Work out the finished part from the listing and answer in its coordinate system (mm). A direction names the side the tool comes from. Round coordinates to 2 decimals unless told otherwise and drop trailing zeros. Write each loop counter-clockwise with the first axis right and the second up, starting at its lowest first coordinate (ties: lowest second). Pieces come first, ordered by that corner, then holes.
1. Determine the mould class of faces 4 (the face through (-29.65, -0.07, 11.31)), 5 (the face through (-20, 0, -1)), 6 (the face through (-10, 0, 5)) for opening direction Y: pulls with the +Y half, pulls with the -Y half, needs draft (parallel to the pull), parting line crosses it, or undercut.
2. Find section C-C (z = 1.25). Write down the section's boundary in (x, y).
3. Flat-ended cylindrical pins translate along their axes: pin 1 Ø6 at (x, y) = (-7.5, 0.5) entering from +Z; pin 2 Ø10 at (y, z) = (-5, 21) entering from +X; pin 3 Ø6 at (x, z) = (-12.5, 1) entering from +Y. Find the tip coordinate at first contact, or state that the pin passes through.
4. Straight lines are drawn through the part: probe 1 along Y at (x, z) = (0, 1.65); probe 2 along X at (y, z) = (3.5, -0.5); probe 3 along Z at (x, y) = (-21.5, 4.25). For each, find the intervals that lie inside material, in ascending order.
5. Find section B-B (y = 0). Write down the section's boundary in (x, z).
6. A tool of negligible diameter and unlimited length cuts with its end or side. For faces 1 (the face through (-2, -6, 0)), 2 (the face through (-24, 0, 15)), 3 (the face through (-26.39, 4.45, 14.86)), from which of +Z, -Z, +X, -X, +Y, -Y can it reach the whole face along a straight path? Write none if from no direction.
7. Find section D-D (z = 22.5). Write down the section's boundary in (x, y), and give its area (3 significant figures).
8. Find section A-A (x = 0). Write down the section's boundary in (y, z).
```python
from build123d import *

# Parameters (mm, degrees)
SKETCH_R      = 8
PAD_DEPTH     = 5
PAD001_DEPTH  = 20
SKETCH002_R   = 10
SKETCH002_R_2 = 6
PAD002_DEPTH  = 2
PAD003_DEPTH  = 2
SKETCH004_R   = 1.65
POCKET_DEPTH  = 27.001


with BuildPart() as part:
    # Sketch → Pad (new body)
    with BuildSketch(Plane.XY):
        with BuildLine():
            ThreePointArc((-2.142857, -9.76771), (10, 0), (-2.142857, 9.76771))
            Line((-28.857143, 3.907084), (-2.142857, 9.76771))
            ThreePointArc((-28.857143, 3.907084), (-32, 0), (-28.857143, -3.907084))
            Line((-2.142857, -9.76771), (-28.857143, -3.907084))
        make_face()
        Circle(SKETCH_R, mode=Mode.SUBTRACT)
    extrude(amount=PAD_DEPTH)

    # Sketch001 (on Face7 of Pad) → Pad001 (join)
    with BuildSketch(Plane.XY.offset(5)):
        with BuildLine():
            ThreePointArc((-28.857143, 3.907084), (-32, -1.3e-05), (-28.857117, -3.90709))
            Line((-24, -4.972619), (-28.857117, -3.90709))
            Line((-24, -4.972619), (-24, 4.972653))
            Line((-24, 4.972653), (-28.857143, 3.907084))
        make_face()
    extrude(amount=PAD001_DEPTH)

    # Sketch002 → Pad002 (join)
    with BuildSketch(Plane(origin=(0, 0, 0), x_dir=(1, 0, 0), z_dir=(0, 0, -1))):
        Circle(SKETCH002_R)
        Circle(SKETCH002_R_2, mode=Mode.SUBTRACT)
    extrude(amount=PAD002_DEPTH)

    # Sketch003 (on Face7 of Pad002) → Pad003 (join)
    with BuildSketch(Plane(origin=(0, 0, 0), x_dir=(1, 0, 0), z_dir=(0, 0, -1))):
        with BuildLine():
            ThreePointArc((-28.857143, 3.907084), (-32, 0), (-28.857143, -3.907084))
            Line((-28.857143, -3.907084), (-22.089875, -5.391699))
            ThreePointArc((-22.089875, -5.391699), (-20, 0), (-22.089875, 5.391699))
            Line((-22.089875, 5.391699), (-28.857143, 3.907084))
        make_face()
    extrude(amount=PAD003_DEPTH)

    # Sketch004 (on Face18 of Pad003) → Pocket (cut, through all)
    with BuildSketch(Plane(origin=(0, 0, -2), x_dir=(1, 0, 0), z_dir=(0, 0, -1))):
        with Locations((-28, 0)):
            Circle(SKETCH004_R)
    extrude(amount=-POCKET_DEPTH, mode=Mode.SUBTRACT)


solid = part.part
```
Worked answers:
1. face 4: undercut
1. face 5: parting line crosses it
1. face 6: needs draft
2. outline: (-28.86, -3.91) - (-2.14, -9.77) arc R10 ccw (long way) to (-2.14, 9.77) - (-28.86, 3.91) arc R4 ccw to start; hole circle Ø3.3 at (-28, 0); hole circle Ø16 at (0, 0)
3. pin 1: stops at z = 5
3. pin 2: stops at x = -24
3. pin 3: stops at y = 8.15
4. probe 1: y = -10 to -8, 8 to 10
4. probe 2: x = -29.94 to -20.81, -9.37 to -4.87, 4.87 to 9.37
4. probe 3: z = -2 to 5
5. outline: (-32, -2) - (-29.65, -2) - (-29.65, 25) - (-32, 25) - close; (-26.35, -2) - (-20, -2) - (-20, 0) - (-10, 0) - (-10, -2) - (-6, -2) - (-6, 0) - (-8, 0) - (-8, 5) - (-24, 5) - (-24, 25) - (-26.35, 25) - close; (6, -2) - (10, -2) - (10, 5) - (8, 5) - (8, 0) - (6, 0) - close
6. face 1: +Z
6. face 2: +Z, +X, +Y, -Y
6. face 3: +Z, -Z, -X, +Y
7. outline: (-28.86, -3.91) - (-24, -4.97) - (-24, 4.97) - (-28.86, 3.91) arc R4 ccw to start; hole circle Ø3.3 at (-28, 0)
7. area: 52.9 mm2
8. outline: (-10, -2) - (-6, -2) - (-6, 0) - (-8, 0) - (-8, 5) - (-10, 5) - close; (6, -2) - (10, -2) - (10, 5) - (8, 5) - (8, 0) - (6, 0) - close
